```python
from build123d import *

# Parameters (mm, degrees)
F0_W     = 31
F0_H     = 105
F1_DEPTH = 10
F2_W     = 20
F2_H     = 99
F3_DEPTH = 10.001
F4_W     = 13
F4_H     = 85
F5_DEPTH = 10.001
F6_SIZE  = 5
F7_R     = 1.7
F8_DEPTH = 105.001
F9_R     = 5


with BuildPart() as f1:
    # F0 (on Right) → F1 (new body)
    with BuildSketch(Plane.YZ):
        with Locations((0.5, 2.5)):
            Rectangle(F0_W, F0_H)
    extrude(amount=F1_DEPTH)

    # F2 (on face) → F3 (cut, through all)
    with BuildSketch(Plane.YZ.offset(10)):
        with Locations((-15, 2.5)):
            Rectangle(F2_W, F2_H)
    extrude(amount=-F3_DEPTH, mode=Mode.SUBTRACT)

    # F4 (on face) → F5 (cut, through all)
    with BuildSketch(Plane.YZ.offset(10)):
        with Locations((1.5, 2.5)):
            Rectangle(F4_W, F4_H)
    extrude(amount=-F5_DEPTH, mode=Mode.SUBTRACT)

    # F6
    f6_edges = [f1.edges().sort_by_distance(p)[0] for p in [
        (5, 16, 55),
        (5, 16, -50),
    ]]
    chamfer(f6_edges, length=F6_SIZE)

    # F7 (on face) → F8 (cut, through all)
    with BuildSketch(Plane.XY.offset(55)):
        with Locations((5, -10)):
            Circle(F7_R)
    extrude(amount=-F8_DEPTH, mode=Mode.SUBTRACT)

    # F9
    f9_edges = [f1.edges().sort_by_distance(p)[0] for p in [
        (5, 8, 45),
        (5, 8, -40),
    ]]
    fillet(f9_edges, radius=F9_R)


solid = f1.part
```
Verification items for the finished model (mm, model axes). A direction names the side the tool comes from. Round coordinates to 2 decimals unless told otherwise and drop trailing zeros. Order: outer loops, then holes, each group sorted by start corner. A loop starts at its lowest first (then second) coordinate and runs counter-clockwise, first axis right, second up. Notation, with made-up numbers: (30.25, 81.5) - (43.25, 81.5) arc R14 ccw to (43.25, 102.5) - close; hole circle Ø6 at (2.5, 68). An arc over 180 degrees is marked (long way). Use CSV: the item, a comma, the result in double quotes. Start each with the question number.
1) Thickness scan on L1, parallel to Z at x = 8.5, y = -6; L2, parallel to Y at x = 5.5, z = 47.5; L3, parallel to Z at x = 1.5, y = -3.5. Record the ranges inside material, lowest first.
2) Section check D-D, the plane x = 4.5. Record the cut outline in (y, z), plus the area to 3 significant figures.
3) Section check C-C, the plane x = 8.5. Record the cut outline in (y, z), plus the area to 3 significant figures.
4) Section check A-A, the plane y = -1. Record the cut outline in (x, z).
5) Mould release check, pull along Y, two halves, no side actions. Record for faces 3 (the flat face through (5, -1, 45)), 4 (the cylindrical face through (5, 7, -38)), 5 (the cylindrical face through (5.8, -11.5, -48.5)): +Y half, -Y half, draft (parallel to the pull), parting line (faces both ways), or undercut.
6) Go/stop test with flat-tipped pins: P1, Ø5, axis at x = 7.5, z = 26, coming from the -Y side; P2, Ø5.5, axis at x = 4.5, z = -44, coming from the -Y side; P3, Ø2, axis at x = 5, y = -10, coming from the -Z side. Record where each tip stops, or that it passes through.
7) Section check B-B, the plane y = -10. Record the cut outline in (x, z).
8) Access from +Z, -Z, +X, -X, +Y, -Y to the whole of each face (thin tool, end or side, straight path). Record for faces 1 (the flat face through (5, -12, 52)), 2 (the flat face through (5, 14, -47)).
Answers:
1,L1,"z = -50 to -47, 52 to 55"
1,L2,"y = -5 to 16"
1,L3,"z = -50 to -40, 45 to 55"
2,outline,"(-15, -50) - (-11.62, -50) - (-11.62, -47) - (-15, -47) - close; (-15, 52) - (-11.62, 52) - (-11.62, 55) - (-15, 55) - close; (-8.38, -50) - (11, -50) - (16, -45) - (16, 50) - (11, 55) - (-8.38, 55) - (-8.38, 52) - (-5, 52) - (-5, 45) - (3, 45) arc R5 cw to (8, 40) - (8, -35) arc R5 cw to (3, -40) - (-5, -40) - (-5, -47) - (-8.38, -47) - close"
2,area,"1,130 mm²"
3,outline,"(-15, -50) - (11, -50) - (16, -45) - (16, 50) - (11, 55) - (-15, 55) - (-15, 52) - (-5, 52) - (-5, 45) - (3, 45) arc R5 cw to (8, 40) - (8, -35) arc R5 cw to (3, -40) - (-5, -40) - (-5, -47) - (-15, -47) - close"
3,area,"1,150 mm²"
4,outline,"(0, -50) - (10, -50) - (10, -40) - (0, -40) - close; (0, 45) - (10, 45) - (10, 55) - (0, 55) - close"
5,face 3,"draft"
5,face 4,"-Y half"
5,face 5,"undercut"
6,P1,"stops at y = 8"
6,P2,"stops at y = -5"
6,P3,"passes through"
7,outline,"(0, -50) - (3.3, -50) - (3.3, -47) - (0, -47) - close; (0, 52) - (3.3, 52) - (3.3, 55) - (0, 55) - close; (6.7, -50) - (10, -50) - (10, -47) - (6.7, -47) - close; (6.7, 52) - (10, 52) - (10, 55) - (6.7, 55) - close"
8,face 1,"+X, -X, -Y"
8,face 2,"-Z, +X, -X, +Y"
